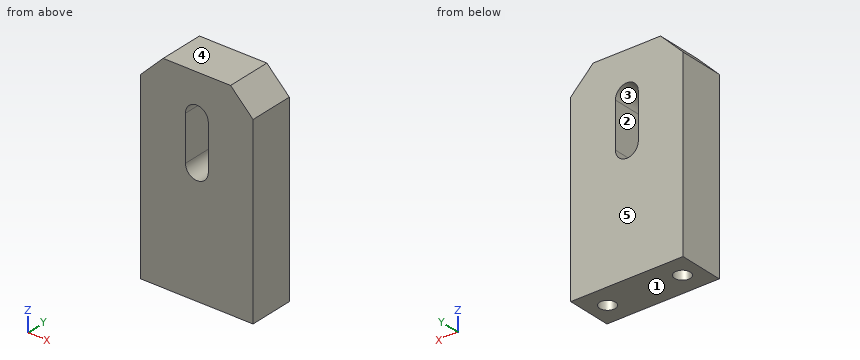
from build123d import *

# Parameters (mm, degrees)
F0_W     = 30
F0_H     = 55
F1_DEPTH = 12
F2_SIZE  = 6
F4_D     = 4.2
F4_DEPTH = 14
F4_TIP   = 1.2618073


with BuildPart() as f1:
    # F0 (on Front) → F1 (new body)
    with BuildSketch(Plane.XZ):
        Rectangle(F0_W, F0_H)
        with BuildLine():
            ThreePointArc((-3.05, 16.5), (0, 19.55), (3.05, 16.5))
            Line((3.05, 16.5), (3.05, 4.5))
            ThreePointArc((3.05, 4.5), (0, 1.45), (-3.05, 4.5))
            Line((-3.05, 4.5), (-3.05, 16.5))
        make_face(mode=Mode.SUBTRACT)
    extrude(amount=F1_DEPTH)

    # F2
    f2_edges = [f1.edges().sort_by_distance(p)[0] for p in [
        (-15, -6, 27.5),
        (15, -6, 27.5),
    ]]
    chamfer(f2_edges, length=F2_SIZE)

    # F4
    with Locations(Plane(origin=(0, 0, -27.5), x_dir=(1, 0, 0), z_dir=(0, 0, -1))):
        with Locations((-10, 6), (10, 6)):
            Hole(F4_D / 2, depth=F4_DEPTH)
            with Locations((0, 0, -(F4_DEPTH + F4_TIP / 2))):  # 118° drill point
                Cone(0, F4_D / 2, F4_TIP, mode=Mode.SUBTRACT)


solid = f1.part
Here's how the part is built. I have some questions about the finished solid (model axes, mm). Face numbers are marked on the shaded views. A direction names the side the tool comes from. Give positions to 0.01 mm unless a question says otherwise; leave off trailing zeros. Loops run counter-clockwise (first coordinate to the right, second up) from the corner with the lowest first, then second, coordinate; pieces in that order, holes last. Notation, with made-up numbers: (37.25, 39.25) -> (52.25, 39.25) arc R14 cw to (52.25, 54.25) -> close; hole circle Ø2 at (70.5, 26.5). An arc over 180 degrees is marked (long way). Answer as a JSON object with one key per item and string values. Group by question number.
Item 1: Thinking about a two-plate mould opening in Z: for the marked faces 3, 4 and 5, which applies, pulls with the +Z half, pulls with the -Z half, needs draft (parallel to the pull), parting line crosses it, or undercut?
Item 2: Imagine slicing it at C-C on z = 11.5. Write out the boundary of the cut face in (x, y), then the cut area to 3 significant figures.
Item 3: Imagine slicing it at B-B on y = -3.25. Write out the boundary of the cut face in (x, z).
Item 4: Imagine slicing it at A-A on x = 0. Write out the boundary of the cut face in (y, z).
Item 5: Imagine slicing it at D-D on z = 23.5. Write out the boundary of the cut face in (x, y), then the cut area to 3 significant figures.
Item 6: On a 3-axis mill with a long thin cutter (end or side, diameter ignored), from which of +Z, -Z, +X, -X, +Y, -Y can I reach the whole of each face in a straight line? I mean the marked faces 1 and 2. Say none if no direction works.
Item 7: I need wall thicknesses on L1, parallel to Y at x = -10, z = -22.5; L2, parallel to X at y = -9.5, z = 13.5; L3, parallel to X at y = -4.5, z = -18. Which ranges of each line are inside material? Lowest first, please.
Answer list:
{
 "1": {"face 3": "undercut", "face 4": "pulls with the +Z half", "face 5": "needs draft"},
 "2": {"outline": "(-15, -12) -> (-3.05, -12) -> (-3.05, 0) -> (-15, 0) -> close; (3.05, -12) -> (15, -12) -> (15, 0) -> (3.05, 0) -> close", "area": "287 mm2"},
 "3": {"outline": "(-15, -27.5) -> (15, -27.5) -> (15, 21.5) -> (9, 27.5) -> (-9, 27.5) -> (-15, 21.5) -> close; hole (-3.05, 4.5) arc R3.05 ccw to (3.05, 4.5) -> (3.05, 16.5) arc R3.05 ccw to (-3.05, 16.5) -> close"},
 "4": {"outline": "(-12, -27.5) -> (0, -27.5) -> (0, 1.45) -> (-12, 1.45) -> close; (-12, 19.55) -> (0, 19.55) -> (0, 27.5) -> (-12, 27.5) -> close"},
 "5": {"outline": "(-13, -12) -> (13, -12) -> (13, 0) -> (-13, 0) -> close", "area": "312 mm2"},
 "6": {"face 1": "-Z, +X, -X, +Y, -Y", "face 2": "+Y, -Y"},
 "7": {"L1": "y = -12 to -8.1, -3.9 to 0", "L2": "x = -15 to -3.05, 3.05 to 15", "L3": "x = -15 to -11.47, -8.53 to 8.53, 11.47 to 15"}
}
